Autodesk Inventor part; units mm, degrees
ref_plane "XZ Plane" through (0, 0, 0) normal (0, 1, 0) x (-1, 0, 0)
sketch "Sketch7" plane through (0, 0, 0) normal (0, 1, 0) x (-1, 0, 0)
  line L0 (0, 0) -> (0, 15.7673)
  line L1 (0, 0) -> (-13.3368, 0) construction
  line L2 (0, 15.7673) -> (-13.3368, 0) construction
  line L3 (0, 15.7673) -> (-18.6413, 0) construction
  line L4 (0, 15.7673) -> (-12.4569, -5.231) construction
  line L5 (0, 0) -> (0, -15.7673)
  line L6 (0, -15.7673) -> (-13.3368, 0) construction
  line L7 (0, -15.7673) -> (-18.6413, 0) construction
  line L8 (0, -15.7673) -> (-12.4569, 5.231) construction
  line L9 (-12.4569, 5.231) -> (-18.6413, 0) construction
  line L10 (-9.3537, 0) -> (-18.5948, -7.8164) construction
  line L11 (-9.3537, 0) -> (-18.0926, 7.3915) construction
  line L12 (0, -29.7093) -> (0, 66.7435)
  line L13 (-53.5, -5.9919) -> (-53.5, 6.008)
  line L14 (17.5786, 0) -> (-94.9714, 0)
  line L15 (-15.989, 2.2434) -> (-10.6846, -2.2434) construction
  line L16 (-10.6846, 2.2434) -> (-15.989, -2.2434) construction
  line L17 (-26.151, -15.9303) -> (-40.3783, -15.9303) construction
  line L18 (-40.3783, -15.9303) -> (-40.3783, -12.7539) construction
  line L19 (-40.3783, -12.7539) -> (-26.151, -12.7539) construction
  line L20 (-26.151, -12.7539) -> (-26.151, -15.9303) construction
  point P0 (-53.5, 0)
  dimension "Roller_Side_difference" = -0.0003
  dimension "d90" = 15.7673
  dimension "d201" = 53.5
  dimension "d343" = 99.548
  dimension "d344" = 99.549
  dimension "d367" = 8.1
sketch "Roller1" plane through (0, 0, 0) normal (0, 1, 0) x (-1, 0, 0)
  line L0 (0, 15.7673) -> (-12.4569, -5.231) construction
  line L1 (0, 15.7673) -> (-18.6413, 0) construction
  line L2 (-9.3537, 0) -> (-18.0926, 7.3915) construction
  line L3 (0, -15.7673) -> (-18.6413, 0) construction
  line L4 (-9.4248, -0.0708) -> (-12.4245, -5.1274)
  line L5 (-12.4245, -5.1274) -> (-18.5445, 0.0491)
  line L6 (-18.5445, 0.0491) -> (-14.0556, 3.846)
  line L7 (-14.0556, 3.846) -> (-9.4248, -0.0708)
  line L8 (-11.7456, 1.8921) -> (-15.4898, -2.5346)
  line L9 (-10.9821, 1.2463) -> (-14.7263, -3.1804)
  point P0 (0, 0)
  point P1 (-15.4845, -2.5391)
  dimension "d345" = 0.025
  dimension "d346" = 0.025
  dimension "d347" = 0.1
  dimension "d348" = 0.1
  dimension "d349" = 99.549
  dimension "d350" = 99.548
  dimension "d357" = 1
  dimension "d369" = 4.0148
sketch "Sketch1" plane through (0, 0, 0) normal (0, 0, 1) x (1, 0, 0)
  circle A0 centre (0, 0) radius 13.3368 construction
  line L0 (0, 0) -> (13.3368, 0)
  line L1 (0, 0) -> (13.3368, 4.025)
  line L2 (13.3368, 0) -> (13.3368, 4.025)
  circle A1 centre (0, 0) radius 53.5
  dimension "d56" = 13.3368
  dimension "d57" = 4.025
  dimension "d400" = 53.5
  dimension "d495" = 2.5
  dimension "d496" = 8
  dimension "d531" = 5.5
  dimension "d532" = 5.5
  dimension "d533" = 5.5
  dimension "d537" = 24.5
  dimension "d538" = 3
  dimension "d543" = 5.5
  dimension "d549" = 3
  dimension "d550" = 3
  dimension "d567" = 5.5
  dimension "d568" = 5.5
sketch "Roller2" plane through (0, 0, 0) normal (0, 1, 0) x (-1, 0, 0)
  line L0 (0, -15.7673) -> (-12.4569, 5.231) construction
  line L1 (-9.3537, 0) -> (-18.5948, -7.8164) construction
  line L2 (0, -15.7673) -> (-18.6413, 0) construction
  line L3 (0, 15.7673) -> (-18.6413, 0) construction
  line L4 (-12.4633, 5.1928) -> (-9.386, 0.0054)
  line L5 (-9.386, 0.0054) -> (-13.9975, -3.8951)
  line L6 (-13.9975, -3.8951) -> (-18.6026, 0)
  line L7 (-18.6026, 0) -> (-12.4633, 5.1928)
  line L8 (-15.533, 2.5964) -> (-11.6918, -1.9449)
  line L9 (-14.7694, 3.2422) -> (-10.9283, -1.2991)
  point P0 (0, 0)
  dimension "d351" = 0.025
  dimension "d352" = 0.025
  dimension "d354" = 0.025
  dimension "d355" = 99.548
  dimension "d356" = 99.549
  dimension "d370" = 0.025
  dimension "d371" = 1
sketch "Sketch22" plane through (0, 0, 0) normal (0, 1, 0) x (-1, 0, 0)
  line L0 (-31.756, 8.0215) -> (-17.5287, 8.0215) construction
  line L1 (-17.5287, 8.0215) -> (-17.5287, 4.8451) construction
  line L2 (-17.5287, 4.8451) -> (-31.756, 4.8451) construction
  line L3 (-31.756, 4.8451) -> (-31.756, 8.0215) construction
  point P0 (0, 0)
  dimension "Roller_Side_difference" = -0.0003
sketch "Sketch2" plane through (0, 0, 0) normal (0, 1, 0) x (-1, 0, 0)
  line L0 (0, 0) -> (0, 13.3368) construction
  line L1 (0, 0) -> (-13.3368, 0)
  line L2 (0, 0) -> (0, -13.3368)
  line L3 (0, -13.3368) -> (-13.3368, 0) construction
  line L4 (0, 13.3368) -> (-13.3368, 0) construction
  line L5 (-78.8928, 52.9645) -> (0, 13.3368) construction
  line L6 (-34.8011, 15.91) -> (0, 13.3368) construction
  line L7 (-34.8011, 15.91) -> (0, -13.3368) construction
  line L8 (-48.3339, 16.9106) -> (0, -13.3368) construction
  point P0 (-17.4708, -4.134)
sketch "Sketch23" plane through (0, 0, 0) normal (0, 1, 0) x (-1, 0, 0)
  line L0 (0, -15.7673) -> (-12.4569, 5.231) construction
  line L1 (0, -15.7673) -> (-18.6413, 0) construction
  line L2 (0, 15.7673) -> (-12.4569, -5.231) construction
  line L3 (-12.4569, 5.231) -> (-18.6413, 0) construction
  line L4 (0, 15.7673) -> (-18.6413, 0) construction
  line L5 (-12.4569, 5.231) -> (-12.4569, -5.231) construction
  line L6 (17.5786, 0) -> (-94.9714, 0)
  line L7 (-11.538, 3.731) -> (-9.3549, 0.051)
  line L8 (-9.3549, -0.051) -> (-11.538, -3.731)
  line L9 (-14.269, 3.731) -> (-18.5898, 0.0764)
  line L10 (-18.5898, -0.0764) -> (-14.269, -3.731)
  arc A0 (-18.5898, 0.0764) -> (-18.5898, -0.0764) centre (-18.5252, 0) ccw
  arc A1 (-9.3549, -0.051) -> (-9.3549, 0.051) centre (-9.4409, 0) ccw
  line L11 (-11.538, 3.731) -> (-11.538, 5.231)
  line L12 (-11.538, 5.231) -> (-1, 5.231)
  line L13 (-1, 5.231) -> (-1, -5.231)
  line L14 (-1, -5.231) -> (-11.538, -5.231)
  line L15 (-11.538, -5.231) -> (-11.538, -3.731)
  line L16 (-14.269, 3.731) -> (-14.269, 5.231)
  line L17 (-14.269, 5.231) -> (-53.5, 5.231)
  line L18 (-53.5, 5.231) -> (-53.5, -5.231)
  line L19 (-14.269, -3.731) -> (-14.269, -5.231)
  line L20 (-14.269, -5.231) -> (-53.5, -5.231)
  line L21 (-12.4569, 5.231) -> (-12.4569, 5.231)
  line L22 (-12.4569, -5.231) -> (-12.4569, -5.231)
  line L23 (0, -29.7093) -> (0, 66.7435)
  line L24 (-18.68, 0) -> (-53.5, 0)
  point P0 (0, 0)
  point P1 (-9.3246, 0)
  point P2 (-18.6252, 0)
  point P3 (-53.5, 0)
  dimension "d378" = 90
  dimension "d379" = 0.1
  dimension "d380" = 0.025
  dimension "d381" = 0.025
  dimension "d382" = 0.025
  dimension "d383" = 0.025
  dimension "d384" = 10.4619
  dimension "d385" = 0
  dimension "d386" = 0
  dimension "d391" = 1
  dimension "d392" = 53.5
  dimension "d393" = 1.5
  dimension "d394" = 1.5
  dimension "d395" = 1.5
  dimension "d396" = 1.5
revolve "RevRoller1" [suppressed]
fillet "Fillet1" [suppressed]
pattern_circular "Circular Pattern13" [suppressed]
feature "Move Body7" [suppressed]
revolve "Revolution13" [suppressed]
fillet "Fillet3" [suppressed]
pattern_circular "Circular Pattern14" [suppressed]
feature "Move Body6" [suppressed]
revolve "Revolution14" add sketch "Sketch23" angle 360 about axis through (0, 0, -10) along (0, 0, 1) contours L13 L14 L15 L8 A1 L6 | L6 A1 L7 L11 L12 L13
ref_plane "Work Plane7" through (0, 0, -25.231) normal (0, 0, -1) x (-1, 0, 0)
sketch "Sketch44" plane through (0, 0, -25.231) normal (0, 0, -1) x (-1, 0, 0)
  circle A0 centre (5, 0) radius 11.538
  line L0 (5, 0) -> (2.5, 0)
  circle A1 centre (2.5, 0) radius 3.5
  point P0 (0, 0)
  dimension "d621" = 2.5
  dimension "d622" = 7
ref_plane "Work Plane8" through (0, 0, -8.607) normal (0, 0, -1) x (-1, 0, 0)
sketch "Sketch45" plane through (0, 0, -8.607) normal (0, 0, -1) x (-1, 0, 0)
  circle A0 centre (5, 0) radius 11.538
  point P0 (0, 0)
loft "Loft1" add profiles "Sketch45" section 1 edges at (-11.538, 0, -5.231)
sketch "Sketch46" plane through (0, 0, 5.231) normal (0, 0, 1) x (1, 0, 0)
  point P0 (0, 0)
extrude "Extrusion39" cut sketch "Sketch44" against normal through all contours A1
ref_plane "Work Plane9" through (50, 0, 0) normal (1, 0, 0) x (0, 1, 0)
sketch "Sketch47" plane through (50, 0, 0) normal (1, 0, 0) x (0, 1, 0)
  line L0 (9.3549, 0.051) -> (-9.3549, 0.051) construction
  circle A0 centre (0, 0) radius 2.75
  circle A1 centre (0, 0) radius 1.5
  line L1 (-1.5877, -2.75) -> (-3.1754, 0)
  line L2 (-3.1754, 0) -> (-1.5877, 2.75)
  line L3 (-1.5877, 2.75) -> (1.5877, 2.75)
  line L4 (1.5877, 2.75) -> (3.1754, 0)
  line L5 (3.1754, 0) -> (1.5877, -2.75)
  line L6 (1.5877, -2.75) -> (-1.5877, -2.75)
  dimension "d626" = 5.5
  dimension "d627" = 3
  dimension "d628" = 5.5
extrude "Extrusion40" [suppressed]
extrude "Extrusion41" [suppressed]
extrude "Extrusion42" [suppressed]
sketch "Sketch40" plane through (0, 0, -5.231) normal (0, 0, -1) x (-1, 0, 0)
  circle A0 centre (53.5, 0) radius 2.75
  circle A1 centre (0, 0) radius 53.5
  point P0 (53.4293, 2.7491)
  point P1 (53.4293, -2.7491)
  dimension "d585" = 8
  dimension "d587" = 1.75
  dimension "d589" = 3
  dimension "d592" = 2
  dimension "d593" = 12
  dimension "d594" = 12
  dimension "d611" = 360
equation "\"Roller_Side_difference\" = -0.001568deg"
equation "\"Cycloid_Top_Plate_Fasner_Inner\" = 61.25"
equation "\"Cycloid_Top_Plate_Fasner_Outer\" = 85.75"
equation "\"Roller_Hole_Radius\" = 1"
equation "\"Distance_To_Bearing\" = 20.65135"
equation "\"d514\" = 0.2"
properties part number "Axle_Printing_TestsRotor_TSB"
Build history of the part. All positions in model axes, mm. A direction names the side the tool comes from. Round coordinates to 2 decimals unless told otherwise and drop trailing zeros. Order: outer loops, then holes, each group sorted by start corner. A loop starts at its lowest first (then second) coordinate and runs counter-clockwise, first axis right, second up. Notation, with made-up numbers: M 4.25,59.5 L 20.25,59.5 A18 ccw 20.25,83.5 Z; hole C -3,74.25 d3. An arc over 180 degrees is marked long. Use CSV: the item, a comma, the result in double quotes. Start each with the question number.
(1) Cut at B-B on z = 2. List the corners of the cut face in (x, y), then the cut area to 3 significant figures.
(2) Flat gauge pins, fed straight in: P1, Ø1.5, axis at x = 5.5, z = 1, coming from the +Y side; P2, Ø8, axis at y = 8, z = 3.5, coming from the +X side; P3, Ø1.5, axis at x = -4.5, z = -2.5, coming from the -Y side. Where does each tip first touch, or does it go through?
(3) Drill centre lines: probe 1 along Y at (x, z) = (0.25, -1); probe 2 along Y at (x, z) = (-2.5, 1.5); probe 3 along Z at (x, y) = (0.5, -9.75). Where is each one in solid material? Low to high.
(4) Tool access for faces 1 (the face through (9.053, -2.851, -0.281)), 2 (the face through (11.005, 3.466, 4.492)), 3 (the face through (-7, 0, -8.607)): list every direction of +Z, -Z, +X, -X, +Y, -Y with a clear straight run to the whole face (end or side of a thin tool).
(5) Cut at A-A on z = 4.25. List the corners of the cut face in (x, y), then the cut area to 3 significant figures.
(6) Mould opens along X. For faces 4 (the face through (2, 0, 5.231)), 5 (the face through (11.005, 3.466, -4.47)), 6 (the face through (1, 0, -2)) say: +X half, -X half, draft (parallel to the pull), parting line (faces both ways), or undercut.
Findings:
1,outline,"C 0,0 d21.02; hole C -2.5,0 d7"
1,area,"309 mm^2"
2,P1,"stops at y = 8.95"
2,P2,"stops at x = 10.82"
2,P3,"stops at y = -10.41"
3,probe 1,"y = -9.91 to -2.17, 2.17 to 9.91"
3,probe 2,"y = -9.9 to -3.5, 3.5 to 9.9"
3,probe 3,"z = -8.61 to -0.74, 0.74 to 5.23"
4,face 1,"none"
4,face 2,"+Z"
4,face 3,"-Z, +X, -X, +Y, -Y"
5,outline,"C 0,0 d23.08; hole C -2.5,0 d7"
5,area,"380 mm^2"
6,face 4,"draft"
6,face 5,"parting line"
6,face 6,"undercut"
